The listing builds one solid part. Answer for the finished solid, in the listing's coordinates (mm). Round coordinates to 2 decimals unless told otherwise and drop trailing zeros. Loops run counter-clockwise (first coordinate to the right, second up) from the corner with the lowest first, then second, coordinate; pieces in that order, holes last. Notation, with made-up numbers: (55.25, 43.25) -> (77.25, 43.25) arc R15 cw to (77.25, 69.25) -> close; hole circle Ø6 at (86, -26.75). An arc over 180 degrees is marked (long way). Write each question's results on one line, items separated by ' | '. Start each with the question number.
(1) The part is cut by section D-D (z = -14). Determine the outline of the cut face in (x, y) (1 decimal), plus the area to 3 significant figures.
(2) Straight lines are drawn through the part: probe 1 along Z at (x, y) = (-152.4, 2); probe 2 along X at (y, z) = (6, 0); probe 3 along Y at (x, z) = (46.5, 4) (3 decimals). For each, find the intervals that lie inside material, in ascending order.
(3) The part is cut by section A-A (z = 0). Determine the outline of the cut face in (x, y) (1 decimal), plus the area to 3 significant figures.
(4) The part is cut by section B-B (y = -1). Determine the outline of the cut face in (x, z).
(5) The part is cut by section C-C (x = -90). Determine the outline of the cut face in (y, z) (1 decimal), plus the area to 3 significant figures.
(6) Flat-ended cylindrical pins translate along their axes: pin 1 (1.5 mm diameter, centred on y = 7.5, z = 18.5, fed in from +X); pin 2 (8 mm diameter, centred on x = 22, z = -19, fed in from +Y) (3 decimals); pin 3 (6 mm diameter, centred on y = 0.5, z = 5, fed in from -X). Find the tip coordinate at first contact, or state that the pin passes through.
```python
from build123d import *
from build123d.topology import SkipClean

# Parameters (mm, degrees)
SKETCH2_R               = 8.0645
BOSS_EXTRUDE2_DEPTH     = 3.175
SKETCH3_R               = 24.1935
SKETCH3_R_2             = 8.0645
BOSS_EXTRUDE3_DEPTH     = 7.9375
CUT_EXTRUDE2_DEPTH      = 181.356612087
CUT_EXTRUDE2_DEPTH_BACK = 181.356612087


with BuildPart() as part:
    # Sketch2 → Boss-Extrude2 (new, symmetric)
    with BuildSketch(Plane(origin=(0, 0, 0), x_dir=(1, 0, 0), z_dir=(0, 1, 0))):
        with BuildLine():
            ThreePointArc((155.790439731, 23.954756536), (0, 34.925), (-155.790439731, 23.954756536))
            ThreePointArc((-155.790439731, 23.954756536), (-176.5935, 0), (-155.790439731, -23.954756536))
            ThreePointArc((-155.790439731, -23.954756536), (0, -34.925), (155.790439731, -23.954756536))
            ThreePointArc((155.790439731, -23.954756536), (176.5935, 0), (155.790439731, 23.954756536))
        make_face()
        with Locations(Location((-152.4, 0, 0), (0, 0, 270))):
            Circle(SKETCH2_R, mode=Mode.SUBTRACT)
        with Locations(Location((152.4, 0, 0), (0, 0, 270))):
            Circle(SKETCH2_R, mode=Mode.SUBTRACT)
    extrude(amount=BOSS_EXTRUDE2_DEPTH, both=True)

    # Sketch3 → Boss-Extrude3 (add)
    with BuildSketch(Plane.XZ.offset(-3.175)):
        with Locations(Location((-152.4, 0, 0), (0, 0, 270))):
            Circle(SKETCH3_R)
        with Locations(Location((-152.4, 0, 0), (0, 0, 270))):
            Circle(SKETCH3_R_2, mode=Mode.SUBTRACT)
    extrude(amount=-BOSS_EXTRUDE3_DEPTH)

    # Sketch2_3 → Cut-Extrude2 (cut, two sides: drawn at the far end of the back side and taken through both)
    with SkipClean():  # the faces are left unmerged after this step: merging them gives an invalid solid
        with BuildSketch(Plane(origin=(0, 0, 0), x_dir=(1, 0, 0), z_dir=(0, 1, 0)).offset(-CUT_EXTRUDE2_DEPTH_BACK)):
            with BuildLine():
                ThreePointArc((-155.790439731, -23.954756536), (0, -34.925), (155.790439731, -23.954756536))
                ThreePointArc((155.790439731, -23.954756536), (154.099417548, -24.133740329), (152.4, -24.1935))
                Line((152.4, -24.1935), (-152.4, -24.1935))
                ThreePointArc((-152.4, -24.1935), (-154.099417548, -24.133740329), (-155.790439731, -23.954756536))
            make_face()
            with BuildLine():
                Line((-152.4, 24.1935), (152.4, 24.1935))
                ThreePointArc((152.4, 24.1935), (154.099417548, 24.133740329), (155.790439731, 23.954756536))
                ThreePointArc((155.790439731, 23.954756536), (0, 34.925), (-155.790439731, 23.954756536))
                ThreePointArc((-155.790439731, 23.954756536), (-154.099417548, 24.133740329), (-152.4, 24.1935))
            make_face()
        extrude(amount=CUT_EXTRUDE2_DEPTH + CUT_EXTRUDE2_DEPTH_BACK, mode=Mode.SUBTRACT)


solid = part.part
```
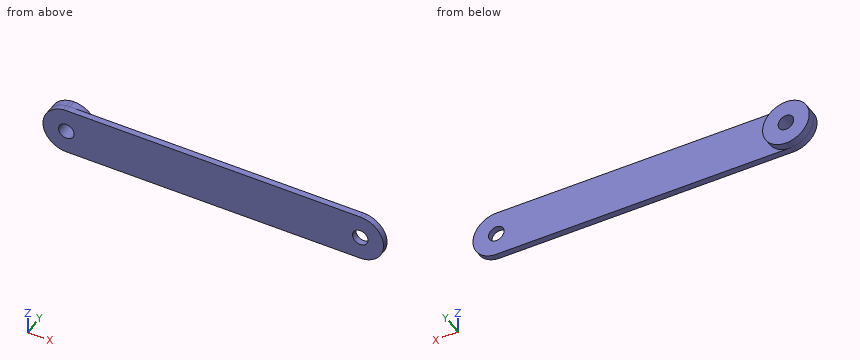
Checked values:
1) outline: (-172.1, -3.2) -> (172.1, -3.2) -> (172.1, 3.2) -> (-132.7, 3.2) -> (-132.7, 11.1) -> (-172.1, 11.1) -> close | area: 2,500 mm2
2) probe 1: z = -24.19 to -8.06, 8.06 to 24.19 | probe 2: x = -176.59 to -160.46, -144.34 to -128.21 | probe 3: y = -3.175 to 3.175
3) outline: (-176.6, -3.2) -> (-160.5, -3.2) -> (-160.5, 11.1) -> (-176.6, 11.1) -> close; (-144.3, -3.2) -> (144.3, -3.2) -> (144.3, 3.2) -> (-128.2, 3.2) -> (-128.2, 11.1) -> (-144.3, 11.1) -> close; (160.5, -3.2) -> (176.6, -3.2) -> (176.6, 3.2) -> (160.5, 3.2) -> close | area: 2,290 mm2
4) outline: (-152.4, -24.19) -> (152.4, -24.19) arc R24.19 ccw to (152.4, 24.19) -> (-152.4, 24.19) arc R24.19 ccw to start; hole circle Ø16.13 at (-152.4, 0); hole circle Ø16.13 at (152.4, 0)
5) outline: (-3.2, -24.2) -> (3.2, -24.2) -> (3.2, 24.2) -> (-3.2, 24.2) -> close | area: 307 mm2
6) pin 1: stops at x = -135.96 | pin 2: stops at y = 3.175 | pin 3: stops at x = -176.51
